Autodesk Inventor part; units mm, degrees
ref_plane "YZ Plane" through (0, 0, 0) normal (1, 0, 0) x (0, 1, 0)
ref_plane "XZ Plane" through (0, 0, 0) normal (0, 1, 0) x (-1, 0, 0)
ref_plane "XY Plane" through (0, 0, 0) normal (0, 0, 1) x (1, 0, 0)
sketch "Sketch1" plane through (0, 0, 0) normal (0, 0, 1) x (1, 0, 0)
  circle A0 centre (0, 0) radius 10.5
  line L0 (0, 0) -> (8, 0)
  circle A1 centre (8, 0) radius 1.25
  circle A2 centre (5.6569, 5.6569) radius 1.25
  circle A3 centre (0, 8) radius 1.25
  circle A4 centre (-5.6569, 5.6569) radius 1.25
  circle A5 centre (-8, 0) radius 1.25
  circle A6 centre (-5.6569, -5.6569) radius 1.25
  circle A7 centre (0, -8) radius 1.25
  circle A8 centre (5.6569, -5.6569) radius 1.25
  dimension "d0" = 21
  dimension "d1" = 8
  dimension "d2" = 2.5
  dimension "d5" = 360
extrude "Extrusion1" add sketch "Sketch1" along normal blind 2
sketch "Sketch2" plane through (0, 0, 2) normal (0, 0, 1) x (1, 0, 0)
  circle A0 centre (0, 0) radius 2.5
  dimension "d9" = 5
extrude "Extrusion3" add sketch "Sketch2" along normal blind 18
sketch "Sketch3" plane through (0, 0, 2) normal (0, 0, 1) x (1, 0, 0)
  circle A0 centre (0, 0) radius 2.5
  circle A1 centre (0, 0) radius 4
  dimension "d14" = 8
extrude "Extrusion4" add sketch "Sketch3" along normal blind 4
properties part number "Drive_shaft2"
CAD build for the part. Positions are in the model's coordinates, mm. A direction names the side the tool comes from. Give positions to 0.01 mm unless a question says otherwise; leave off trailing zeros. Loops run counter-clockwise (first coordinate to the right, second up) from the corner with the lowest first, then second, coordinate; pieces in that order, holes last. Notation, with made-up numbers: M -28,83.25 L -14,83.25 A27 cw -14,115.25 Z; hole C 73,55.25 d10. An arc over 180 degrees is marked long. Answer in a Markdown table with one row per item. Add a question column.
Item 1: Tool access for faces 1 (the face through (-6.65, -4.9, 0.99)), 2 (the face through (2, 2, 6)): list every direction of +Z, -Z, +X, -X, +Y, -Y with a clear straight run to the whole face (end or side of a thin tool).
Item 2: Band-saw the part on D-D on z = 8.25. Give the cut face in (x, y).
Item 3: Band-saw the part on B-B on x = -5. Give the cut face in (y, z).
Item 4: Drop flat-ended pins along their axis: P1, Ø5, axis at y = 4, z = 15, coming from the +X side; P2, Ø3, axis at x = 7.5, y = 3.5, coming from the -Z side; P3, Ø2, axis at x = 0, y = 8, coming from the +Z side; P4, Ø3, axis at x = 0, y = -8, coming from the +Z side. Give the stop position or say it passes through.
Item 5: Probe probe 1 along Z at (x, y) = (3.5, 2); probe 2 along Y at (x, z) = (2, 10.75); probe 3 along Y at (x, z) = (0.5, 14). List the from-to ranges inside material, lowest first.
Item 6: Band-saw the part on A-A on y = 8. Give the cut face in (x, z).
Reply:
| question | item | result |
|---|---|---|
| 1 | face 1 | +Z, -Z |
| 1 | face 2 | +Z |
| 2 | outline | C 0,0 d5 |
| 3 | outline | M -9.23,0 L -6.72,0 L -6.72,2 L -9.23,2 Z; M -4.59,0 L 4.59,0 L 4.59,2 L -4.59,2 Z; M 6.72,0 L 9.23,0 L 9.23,2 L 6.72,2 Z |
| 4 | P1 | stops at x = 2 |
| 4 | P2 | stops at z = 0 |
| 4 | P3 | passes through |
| 4 | P4 | stops at z = 2 |
| 5 | probe 1 | z = 0 to 2 |
| 5 | probe 2 | y = -1.5 to 1.5 |
| 5 | probe 3 | y = -2.45 to 2.45 |
| 6 | outline | M -6.8,0 L -1.25,0 L -1.25,2 L -6.8,2 Z; M 1.25,0 L 6.8,0 L 6.8,2 L 1.25,2 Z |
